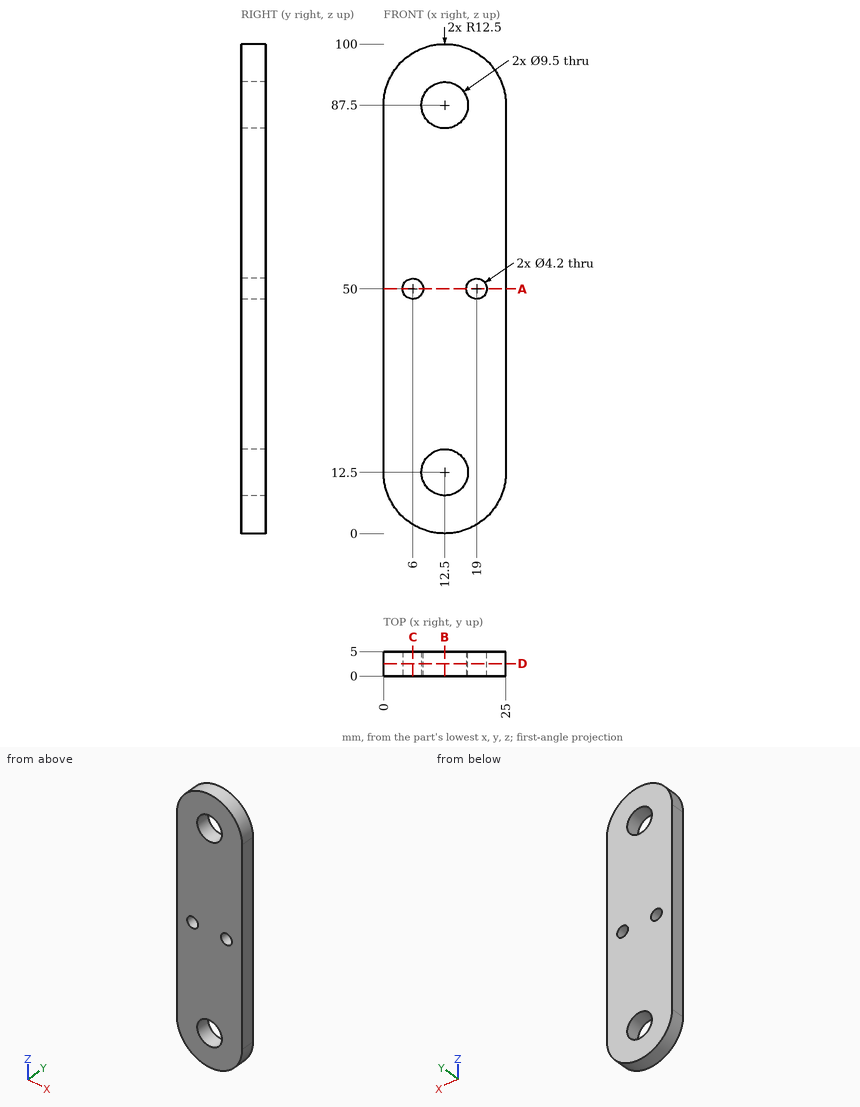
Study the drawing (mm; zero at the part's minimum x, y, z) and answer. Round coordinates to 2 decimals unless told otherwise and drop trailing zeros. Loops run counter-clockwise (first coordinate to the right, second up) from the corner with the lowest first, then second, coordinate; pieces in that order, holes last. Notation, with made-up numbers: (52.5, 79) -> (86.5, 79) arc R14 ccw to (86.5, 87) -> close; hole circle Ø3 at (-18.75, -14). An arc over 180 degrees is marked (long way). One line per item, written item: value.
1) A cutting plane is placed at D-D (y = 2.55). Determine the outline of the cut face in (x, z).
Answer list:
outline: (0, 12.5) arc R12.5 ccw to (25, 12.5) -> (25, 87.5) arc R12.5 ccw to (0, 87.5) -> close; hole circle Ø4.2 at (6, 50); hole circle Ø9.5 at (12.5, 12.5); hole circle Ø9.5 at (12.5, 87.5); hole circle Ø4.2 at (19, 50)
2) A cutting plane is placed at B-B (x = 12.5). Determine the outline of the cut face in (y, z).
Answer list:
outline: (0, 0) -> (5, 0) -> (5, 7.75) -> (0, 7.75) -> close; (0, 17.25) -> (5, 17.25) -> (5, 82.75) -> (0, 82.75) -> close; (0, 92.25) -> (5, 92.25) -> (5, 100) -> (0, 100) -> close
3) Consider L1, parallel to Z at x = 12.5, y = 1.1; L2, parallel to X at y = 1.6, z = 50; L3, parallel to X at y = 2.05, z = 87.5. Determine where each line is inside the solid, lowest interval first. Write a range as [from, to].
Answer list:
L1: z = [0, 7.75], [17.25, 82.75], [92.25, 100]
L2: x = [0, 3.9], [8.1, 16.9], [21.1, 25]
L3: x = [0, 7.75], [17.25, 25]
4) Flat-ended cylindrical pins translate along their axes: P1, Ø15, axis at x = 12.5, z = 87.5, coming from the +Y side; P2, Ø8.5, axis at x = 12.5, z = 12.5, coming from the +Y side. Find the tip coordinate at first contact, or state that the pin passes through.
Answer list:
P1: stops at y = 5
P2: passes through
5) A cutting plane is placed at A-A (z = 50). Determine the outline of the cut face in (x, y).
Answer list:
outline: (0, 0) -> (3.9, 0) -> (3.9, 5) -> (0, 5) -> close; (8.1, 0) -> (16.9, 0) -> (16.9, 5) -> (8.1, 5) -> close; (21.1, 0) -> (25, 0) -> (25, 5) -> (21.1, 5) -> close
6) A cutting plane is placed at C-C (x = 6). Determine the outline of the cut face in (y, z), and give its area (3 significant figures).
Answer list:
outline: (0, 1.82) -> (5, 1.82) -> (5, 47.9) -> (0, 47.9) -> close; (0, 52.1) -> (5, 52.1) -> (5, 98.18) -> (0, 98.18) -> close
area: 461 mm²
